Autodesk Fusion 360 part; units mm, degrees
sketch "Sketch1" plane through (0, 0, 0) normal (0, 0, 1) x (1, 0, 0)
  line L0 (-90, 40) -> (90, 40)
  line L1 (90, 40) -> (90, -40)
  line L2 (90, -40) -> (-90, -40)
  line L3 (-90, -40) -> (-90, 40)
  line L4 (-90, 40) -> (90, -40) construction
  line L5 (90, 40) -> (-90, -40) construction
  circle A0 centre (-25, 22.3325) radius 5.5
  circle A1 centre (-75, 22.3727) radius 5.5
  circle A2 centre (-25.3826, -22.6675) radius 5.5
  circle A3 centre (75, 22.1737) radius 5.5
  circle A4 centre (25, 22.2838) radius 5.5
  circle A5 centre (-75.3826, -22.6273) radius 5.5
  circle A6 centre (24.6174, -22.7162) radius 5.5
  circle A7 centre (74.6174, -22.8263) radius 5.5
  circle A8 centre (0, 0) radius 7
  point P0 (-90, 40)
  point P1 (-24.0015, 35.2175)
  dimension "d1" = 80
  dimension "d2" = 180
  dimension "d3" = 11
  dimension "d4" = 11
  dimension "d5" = 11
  dimension "d7" = 11
  dimension "d8" = 11
  dimension "d9" = 11
  dimension "d11" = 11
  dimension "d12" = 11
  dimension "d15" = 50
  dimension "d16" = 50
  dimension "d17" = 50
  dimension "d18" = 50
  dimension "d19" = 50
  dimension "d20" = 50
  dimension "d21" = 45
  dimension "d22" = 45
  dimension "d23" = 45
  dimension "d25" = 45
  dimension "d26" = 14
extrude "Extrude1" add sketch "Sketch1" along normal blind 7
sketch "Sketch3" plane through (0, 0, 7) normal (0, 0, 1) x (-1, 0, 0)
  circle A0 centre (75.3826, 22.6273) radius 5.5
  circle A1 centre (-74.6174, 22.8263) radius 5.5
  circle A2 centre (0, 0) radius 7
  circle A3 centre (75, -22.3727) radius 5.5
  circle A4 centre (25, -22.3325) radius 5.5
  circle A5 centre (-75, -22.1737) radius 5.5
  circle A6 centre (-24.6174, 22.7162) radius 5.5
  circle A7 centre (-25, -22.2838) radius 5.5
  circle A8 centre (25.3826, 22.6675) radius 5.5
  line L0 (90, 40) -> (-90, 40)
  line L1 (-90, 40) -> (-90, -40)
  line L2 (-90, -40) -> (90, -40)
  line L3 (90, -40) -> (90, 40)
  circle A9 centre (0, -31) radius 2
  line L4 (-20, 0) -> (-2.5, 0)
  circle A10 centre (0, 31) radius 2
  dimension "d29" = 4
  dimension "d30" = 31
extrude "Extrude2" cut sketch "Sketch3" against normal blind 14 contours A9 | A10
extrude "Extrude3" cut 1 faces at (-43.1381, 6.099, 7) along direction (0, 0, -1) blind 4
equation "d30 = 27 mm + 4 mm"
Design review of the part built by this model. Coordinates are the model's own, in mm. Coordinates: 2 decimals unless noted, no trailing zeros. Loops run counter-clockwise (first coordinate to the right, second up) from the corner with the lowest first, then second, coordinate; pieces in that order, holes last. Notation, with made-up numbers: (44.5, 33) - (103.5, 33) arc R23 ccw to (103.5, 41) - close; hole circle Ø7 at (24, 74). An arc over 180 degrees is marked (long way). Use CSV: the item, a comma, the result in double quotes. Start each with the question number.
1) The part is to be moulded in two halves that separate along X. For faces 1 (the flat face through (90, 1, 1)), 2 (the cylindrical face through (-19.754, 20.68, 1.479)), 3 (the flat face through (-1, 9, 3)), say which applies: +X half, -X half, draft (parallel to the pull), parting line (faces both ways), or undercut.
2) For pin 1 Ø10 at (x, y) = (25, 22.28) entering from -Z, flat-tipped, find the tip position at first contact; note if it passes through.
3) Wall thickness on L1, parallel to Y at x = -25, z = 0.9; L2, parallel to Y at x = 75, z = 0.85; L3, parallel to X at y = -22.5, z = 0.65: over which ranges is each line inside the solid? List them lowest first. Write a range as from..to.
4) Consider section C-C on x = 71.5. Write out the cut boundary in (y, z).
5) Consider section A-A on x = 0. Write out the cut boundary in (y, z).
6) Consider section B-B on y = -31. Write out the cut boundary in (x, z), then the cut area to 3 significant figures.
7) Consider section D-D on z = 1.7. Give the number of separate pieces and of enclosed holes in the cut face, then the cut area to 3 significant figures.
Geometry says:
1,face 1,"+X half"
1,face 2,"undercut"
1,face 3,"draft"
2,pin 1,"through"
3,L1,"-40..-28.15, -17.18..16.83, 27.83..40"
3,L2,"-40..-28.31, -17.34..16.67, 27.67..40"
3,L3,"-90..-80.88, -69.88..-30.88, -19.89..19.12, 30.11..69.13, 80.11..90"
4,outline,"(-40, 0) - (-27.36, 0) - (-27.36, 3) - (-40, 3) - close; (-18.3, 0) - (17.93, 0) - (17.93, 3) - (-18.3, 3) - close; (26.42, 0) - (40, 0) - (40, 3) - (26.42, 3) - close"
5,outline,"(-40, 0) - (-33, 0) - (-33, 3) - (-40, 3) - close; (-29, 0) - (-7, 0) - (-7, 3) - (-29, 3) - close; (7, 0) - (29, 0) - (29, 3) - (7, 3) - close; (33, 0) - (40, 0) - (40, 3) - (33, 3) - close"
6,outline,"(-90, 0) - (-2, 0) - (-2, 3) - (-90, 3) - close; (2, 0) - (90, 0) - (90, 3) - (2, 3) - close"
6,area,"528 mm^2"
7,separate pieces,"1"
7,enclosed holes,"11"
7,area,"13,500 mm^2"
